```python
from build123d import *

# Parameters (mm, degrees)
SKETCH1_W           = 748
SKETCH1_H           = 180
SKETCH1_R           = 2.5
SKETCH1_R_2         = 6
BOSS_EXTRUDE1_DEPTH = 4


with BuildPart() as part:
    # Sketch1 → Boss-Extrude1 (new body)
    with BuildSketch(Plane(origin=(0, 0, 0), x_dir=(1, 0, 0), z_dir=(0, 1, 0))):
        Rectangle(SKETCH1_W, SKETCH1_H)
        with Locations((-344, 80)):
            Circle(SKETCH1_R, mode=Mode.SUBTRACT)
        with Locations((0, 80)):
            Circle(SKETCH1_R, mode=Mode.SUBTRACT)
        with Locations((344, 80)):
            Circle(SKETCH1_R, mode=Mode.SUBTRACT)
        with Locations((-344, -80)):
            Circle(SKETCH1_R, mode=Mode.SUBTRACT)
        with Locations((0, -80)):
            Circle(SKETCH1_R, mode=Mode.SUBTRACT)
        with Locations((344, -80)):
            Circle(SKETCH1_R, mode=Mode.SUBTRACT)
        with Locations((-360, 80)):
            Circle(SKETCH1_R_2, mode=Mode.SUBTRACT)
        with Locations((-360, -80)):
            Circle(SKETCH1_R_2, mode=Mode.SUBTRACT)
        with Locations((360, -80)):
            Circle(SKETCH1_R_2, mode=Mode.SUBTRACT)
        with Locations((360, 80)):
            Circle(SKETCH1_R_2, mode=Mode.SUBTRACT)
    extrude(amount=BOSS_EXTRUDE1_DEPTH)


solid = part.part
```
Input: part model. Units: mm. Frame: model coordinates. Give positions to 0.01 mm unless a question says otherwise; leave off trailing zeros. Use a Markdown table: item, result.
Q1. First-contact query: P1, Ø11, axis at x = -360, z = -80, coming from the +Y side. Flat tip, straight axial feed; report the tip coordinate or a pass-through.
Entries:
| item | result |
|---|---|
| P1 | passes through |
Q2. Pull-direction query (Z, two-part tool) for faces 1 (the cylindrical face through (-354.277, 1.972, 78.198)), 2 (the cylindrical face through (-354.277, 1.972, -81.802)), 3 (the flat face through (-5, 4, -1)); classes: pulls with the +Z half, pulls with the -Z half, needs draft (parallel to the pull), parting line crosses it, or undercut.
Entries:
| item | result |
|---|---|
| face 1 | undercut |
| face 2 | undercut |
| face 3 | needs draft |
Q3. Ray query, probe 1 along X at (y, z) = (1, 80); probe 2 along Z at (x, y) = (0, 1.8); probe 3 along Z at (x, y) = (-360, 1.3). Return the intervals inside material, ascending. Write a range as from..to.
Entries:
| item | result |
|---|---|
| probe 1 | x = -374..-366, -354..-346.5, -341.5..-2.5, 2.5..341.5, 346.5..354, 366..374 |
| probe 2 | z = -90..-82.5, -77.5..77.5, 82.5..90 |
| probe 3 | z = -90..-86, -74..74, 86..90 |
